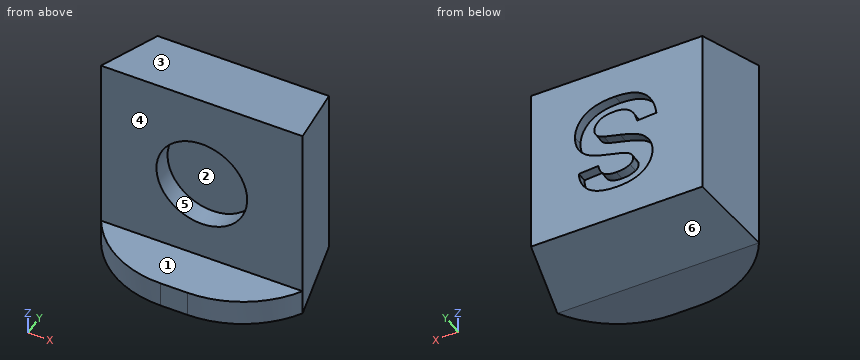
```python
from build123d import *

# Parameters (mm, degrees)
SKETCH1_W               = 8
SKETCH1_H               = 8
BOSS_EXTRUDE1_DEPTH     = 3
CUT_EXTRUDE1_DEPTH      = 12.704699911
CUT_EXTRUDE1_DEPTH_BACK = 12.704699911
CUT_EXTRUDE2_DEPTH      = 11
SKETCH4_R               = 1.8
CUT_EXTRUDE3_DEPTH      = 0.8
SKETCH5_W               = 8
SKETCH5_H               = 1
BOSS_EXTRUDE2_DEPTH     = 2
FILLET1_R               = 4
CUT_EXTRUDE4_DEPTH      = 0.4


with BuildPart() as part:
    # Sketch1 → Boss-Extrude1 (new body)
    with BuildSketch(Plane(origin=(0, 0, 0), x_dir=(1, 0, 0), z_dir=(0, 1, 0))):
        with Locations((4, 4)):
            Rectangle(SKETCH1_W, SKETCH1_H)
    extrude(amount=BOSS_EXTRUDE1_DEPTH)

    # Sketch2 → Cut-Extrude1 (cut, two sides: drawn at the far end of the back side and taken through both)
    with BuildSketch(Plane.XY.offset(-CUT_EXTRUDE1_DEPTH_BACK)):
        Polygon((0, 0), (0.6, 3), (0, 3), align=None)
        Polygon((8, 0), (7.4, 3), (8, 3), align=None)
    extrude(amount=CUT_EXTRUDE1_DEPTH + CUT_EXTRUDE1_DEPTH_BACK, mode=Mode.SUBTRACT)

    # Sketch3 → Cut-Extrude2 (cut)
    with BuildSketch(Plane(origin=(0, 0, 0), x_dir=(0, 0, -1), z_dir=(1, 0, 0))):
        Polygon((0, 0), (0.6, 3), (0, 3), align=None)
        Polygon((8, 3), (7.4, 3), (8, 0), align=None)
    extrude(amount=CUT_EXTRUDE2_DEPTH, mode=Mode.SUBTRACT)

    # Sketch4 → Cut-Extrude3 (cut)
    with BuildSketch(Plane.XZ):
        with Locations(Location((4, -3.75, 0), (0, 0, 270))):
            Circle(SKETCH4_R)
    extrude(amount=-CUT_EXTRUDE3_DEPTH, mode=Mode.SUBTRACT)

    # Sketch5 → Boss-Extrude2 (add)
    with BuildSketch(Plane.XZ):
        with Locations((4, -7.5)):
            Rectangle(SKETCH5_W, SKETCH5_H)
    extrude(amount=BOSS_EXTRUDE2_DEPTH)

    # Fillet1
    # the kernel refuses this fillet: 4 mm, written as the material it takes off along each edge
    with BuildSketch(Plane(origin=(8, -2, -16.660254038), x_dir=(0, 1, 0), z_dir=(0, 0, 1)), Plane(origin=(0, -2, 1.660254038), x_dir=(0, 1, 0), z_dir=(0, 0, -1))) as fillet1_piece_1:
        with BuildLine():
            CenterArc((4, 3.464101615), FILLET1_R, 180, 60)
            Line((0, 3.464101615), (-0.08, 3.464101615))
            Line((-0.08, 3.464101615), (-0.08, 0))
            Line((-0.08, 0), (0, -0.08))
            ThreePointArc((0, -0.08), (1, -0.08), (1.96, -0.069282032))
            Line((1.96, -0.069282032), (2, 0))
        make_face()
    extrude(amount=18.320508076, mode=Mode.SUBTRACT)

    # Sketch6 → Cut-Extrude4 (cut)
    with BuildSketch(Plane(origin=(0, 3, 0), x_dir=(1, 0, 0), z_dir=(0, 1, 0))):
        with BuildLine():
            Line((2.423916505, 3.336189685), (3.193147274, 3.387471736))
            add(Edge.make_bspline(
                [(3.193147274, 3.387471736), (3.199275518, 3.35528983), (3.211179242, 3.292778523), (3.237627081, 3.203691377), (3.266738832, 3.12063689), (3.30152897, 3.044505684), (3.339615284, 2.973890515), (3.38412658, 2.910803039), (3.431957638, 2.853229033), (3.485476185, 2.803236311), (3.543783948, 2.759451994), (3.607171876, 2.722111271), (3.674953108, 2.6897922), (3.747293374, 2.663178469), (3.824938253, 2.64331119), (3.907211345, 2.629176798), (3.994230643, 2.620125524), (4.053701404, 2.618879435), (4.084172915, 2.618240967)],
                knots=[0, 0, 0, 0, 1.204560339, 2.339781841, 3.415289417, 4.440034832, 5.416475564, 6.362424008, 7.275913008, 8.16578645, 9.05021719, 9.95355393, 10.867835453, 11.809845306, 12.784702352, 13.812224031, 14.87903166, 16, 16, 16, 16], degree=3))
            add(Edge.make_bspline(
                [(4.084172915, 2.618240967), (4.116246108, 2.618590883), (4.178630121, 2.619271489), (4.269031453, 2.627715), (4.353560804, 2.639811238), (4.431471751, 2.6589593), (4.504219207, 2.680373377), (4.569996427, 2.709670116), (4.629867843, 2.743459668), (4.683679212, 2.781802056), (4.730640445, 2.824326515), (4.771724475, 2.86872067), (4.807505951, 2.914025405), (4.835668504, 2.962251146), (4.858460082, 3.011447443), (4.873523718, 3.063081907), (4.883700097, 3.1159689), (4.884867031, 3.152113555), (4.885454967, 3.1703243)],
                knots=[0, 0, 0, 0, 1.417779877, 2.757654889, 4.012140507, 5.189587551, 6.302846416, 7.360586765, 8.365575446, 9.33904572, 10.275781718, 11.161696098, 12.012180333, 12.822428111, 13.625933072, 14.403138519, 15.195454004, 16, 16, 16, 16], degree=3))
            add(Edge.make_bspline(
                [(4.885454967, 3.1703243), (4.884733913, 3.193140887), (4.883323278, 3.237778199), (4.866340641, 3.301592127), (4.840872442, 3.360713887), (4.802526135, 3.41427025), (4.750979261, 3.463212961), (4.685226085, 3.508997669), (4.603431212, 3.550186), (4.542750055, 3.573160928), (4.510454967, 3.585388403)],
                knots=[0, 0, 0, 0, 0.90494901, 1.770400303, 2.607161909, 3.452839393, 4.36912122, 5.420987164, 6.627424851, 8, 8, 8, 8], degree=3))
            add(Edge.make_bspline(
                [(4.510454967, 3.585388403), (4.496597999, 3.590031937), (4.465588357, 3.600423411), (4.4126892, 3.615282239), (4.348970759, 3.633836968), (4.273512264, 3.654927379), (4.186339087, 3.676497317), (4.088424838, 3.703069034), (3.978575834, 3.729510064), (3.901725338, 3.749028827), (3.861416505, 3.759266608)],
                knots=[0, 0, 0, 0, 0.521821638, 1.167752076, 1.961721917, 2.891982557, 3.96540661, 5.168436773, 6.514817513, 8, 8, 8, 8], degree=3))
            add(Edge.make_bspline(
                [(3.861416505, 3.759266608), (3.808922441, 3.772373151), (3.707643728, 3.797660082), (3.563197092, 3.84264374), (3.430159098, 3.887337495), (3.309810688, 3.935832618), (3.200824367, 3.984842463), (3.104963023, 4.037807847), (3.02022624, 4.091978089), (2.970848149, 4.132466251), (2.947153685, 4.151894813)],
                knots=[0, 0, 0, 0, 1.293880989, 2.496331788, 3.617634808, 4.64976062, 5.598842568, 6.473791081, 7.267636666, 8, 8, 8, 8], degree=3))
            add(Edge.make_bspline(
                [(2.947153685, 4.151894813), (2.917769469, 4.179407128), (2.860158996, 4.233347566), (2.784323751, 4.321982057), (2.720601495, 4.415610216), (2.668151102, 4.513540942), (2.627765291, 4.616338017), (2.599140348, 4.723313361), (2.580613245, 4.834746169), (2.578722682, 4.91063455), (2.577762659, 4.949170454)],
                knots=[0, 0, 0, 0, 1.064429417, 2.086912298, 3.078678339, 4.055528992, 5.020032834, 5.993708893, 6.981211098, 8, 8, 8, 8], degree=3))
            add(Edge.make_bspline(
                [(2.577762659, 4.949170454), (2.579632311, 4.999035454), (2.583341142, 5.097952729), (2.617353538, 5.24334762), (2.670335558, 5.383642492), (2.731782138, 5.495041815), (2.790819043, 5.579315825), (2.839844896, 5.639790083), (2.893704531, 5.696388175), (2.953135712, 5.747729494), (3.015931612, 5.796821395), (3.084525186, 5.840415592), (3.156971597, 5.881478913), (3.261809808, 5.93015757), (3.404151332, 5.980885512), (3.589345301, 6.023645948), (3.790984862, 6.049350493), (3.930782191, 6.052503897), (4.003243428, 6.054138403)],
                knots=[0, 0, 0, 0, 1.180131776, 2.341029169, 3.518901375, 4.725685298, 5.343762192, 5.955650671, 6.568945152, 7.192346361, 7.815201106, 8.455999361, 9.116257477, 9.787318263, 11.192748436, 12.688084276, 14.283332633, 16, 16, 16, 16], degree=3))
            add(Edge.make_bspline(
                [(4.003243428, 6.054138403), (4.062574751, 6.053344994), (4.177972905, 6.051801831), (4.345255933, 6.036197125), (4.501507358, 6.011910245), (4.646178875, 5.977046542), (4.779337891, 5.930982439), (4.901500568, 5.876111383), (5.012563098, 5.81096567), (5.111173405, 5.735171454), (5.199025737, 5.651613191), (5.275662846, 5.560343317), (5.341377732, 5.462514514), (5.396594511, 5.358198276), (5.439956101, 5.246858263), (5.471803478, 5.128633406), (5.492867609, 5.003801978), (5.498147397, 4.918266237), (5.500839582, 4.874651223)],
                knots=[0, 0, 0, 0, 1.325124071, 2.577337985, 3.749592149, 4.855247722, 5.896868755, 6.892903601, 7.842551483, 8.766257401, 9.665194363, 10.546067736, 11.423174165, 12.293291263, 13.177512979, 14.086532529, 15.024315359, 16, 16, 16, 16], degree=3))
            Line((5.500839582, 4.874651223), (4.731608813, 4.823369172))
            add(Edge.make_bspline(
                [(4.731608813, 4.823369172), (4.727171315, 4.847490186), (4.718523093, 4.894499533), (4.699719489, 4.96182647), (4.678509937, 5.024096207), (4.653685255, 5.081308344), (4.623700039, 5.13243816), (4.591067506, 5.179094223), (4.554887475, 5.220654869), (4.51396201, 5.255982033), (4.469697485, 5.288128305), (4.419251527, 5.313894286), (4.364737876, 5.337799444), (4.30408262, 5.355770261), (4.238450559, 5.370025359), (4.167803464, 5.380593162), (4.091994892, 5.385752959), (4.039841388, 5.386885694), (4.012858813, 5.387471736)],
                knots=[0, 0, 0, 0, 1.151066407, 2.24330871, 3.278475654, 4.238599069, 5.165719782, 6.056502506, 6.909492653, 7.744782051, 8.590364415, 9.471203867, 10.39832458, 11.382154319, 12.435022857, 13.550631277, 14.73277401, 16, 16, 16, 16], degree=3))
            add(Edge.make_bspline(
                [(4.012858813, 5.387471736), (3.984804304, 5.386954358), (3.930223002, 5.385947775), (3.850683499, 5.379770524), (3.776069477, 5.368367912), (3.706014485, 5.353524542), (3.640612102, 5.333331162), (3.580000346, 5.308708643), (3.523901913, 5.279720359), (3.489695535, 5.256913378), (3.47279471, 5.245644813)],
                knots=[0, 0, 0, 0, 1.186678824, 2.308736671, 3.37120409, 4.377216403, 5.334874112, 6.262130804, 7.141346615, 8, 8, 8, 8], degree=3))
            add(Edge.make_bspline(
                [(3.47279471, 5.245644813), (3.453453136, 5.230251633), (3.415994509, 5.200439822), (3.3756811, 5.141243702), (3.351412335, 5.074383458), (3.348491314, 5.027102037), (3.346993428, 5.002856352)],
                knots=[0, 0, 0, 0, 1.037857257, 2.010007357, 2.979541333, 4, 4, 4, 4], degree=3))
            add(Edge.make_bspline(
                [(3.346993428, 5.002856352), (3.348218426, 4.980197149), (3.350631475, 4.935562125), (3.374970191, 4.872157107), (3.41239982, 4.813407798), (3.447371668, 4.781494404), (3.465583172, 4.764875582)],
                knots=[0, 0, 0, 0, 0.98538058, 1.941042925, 2.927803204, 4, 4, 4, 4], degree=3))
            add(Edge.make_bspline(
                [(3.465583172, 4.764875582), (3.480036346, 4.754089134), (3.512333176, 4.72998591), (3.571494566, 4.699348433), (3.642903916, 4.666166195), (3.728189187, 4.633726893), (3.826783574, 4.601347807), (3.938693075, 4.567540299), (4.063986517, 4.533278892), (4.199470233, 4.500098399), (4.337024364, 4.467483879), (4.46828848, 4.431827004), (4.590345232, 4.397064309), (4.702628677, 4.360627363), (4.805717615, 4.325156109), (4.899111277, 4.288724577), (4.98345094, 4.253244341), (5.081800337, 4.204456503), (5.193269487, 4.138371404), (5.310101731, 4.042305693), (5.413424942, 3.934321559), (5.485417809, 3.83249997), (5.534873142, 3.744930694), (5.566717158, 3.675127784), (5.59426473, 3.601573118), (5.616688379, 3.524185412), (5.632940128, 3.442855773), (5.646389397, 3.358205559), (5.653260877, 3.269531733), (5.654205671, 3.209062493), (5.654685736, 3.178337121)],
                knots=[0, 0, 0, 0, 0.511875881, 1.143829537, 1.88775736, 2.750598373, 3.734912702, 4.837306479, 6.073130119, 7.42648979, 8.801963576, 10.091065733, 11.292408984, 12.408830014, 13.446061236, 14.39066453, 15.257936293, 16.045629259, 17.510392066, 18.929669597, 20.331293837, 21.746891395, 22.460690638, 23.187651344, 23.925159671, 24.69163991, 25.474819891, 26.281170188, 27.126635539, 28, 28, 28, 28], degree=3))
            add(Edge.make_bspline(
                [(5.654685736, 3.178337121), (5.654025632, 3.150001459), (5.652714728, 3.093729578), (5.643553782, 3.010207902), (5.629386607, 2.928169417), (5.608414322, 2.847511277), (5.580592445, 2.768392154), (5.549267222, 2.689670139), (5.510096795, 2.613061996), (5.465515506, 2.538504273), (5.41634032, 2.466052922), (5.360615699, 2.3992182), (5.301614691, 2.335770341), (5.235567289, 2.279262071), (5.166552067, 2.225117883), (5.091412341, 2.177166881), (5.011908526, 2.133775469), (4.927537931, 2.095267608), (4.838001417, 2.061711489), (4.743415274, 2.031844209), (4.642927337, 2.007400135), (4.537375532, 1.986448484), (4.426373586, 1.970515295), (4.310060277, 1.959390224), (4.188409162, 1.953116354), (4.105547428, 1.952094705), (4.063339582, 1.9515743)],
                knots=[0, 0, 0, 0, 0.900570041, 1.788444861, 2.667795364, 3.545012114, 4.433698372, 5.332345486, 6.235991676, 7.164928091, 8.092777575, 9.015680987, 9.928493428, 10.842962589, 11.775229507, 12.714851019, 13.672254427, 14.652424454, 15.660007982, 16.709910502, 17.803296389, 18.945495772, 20.129342395, 21.366102753, 22.658353839, 24, 24, 24, 24], degree=3))
            add(Edge.make_bspline(
                [(4.063339582, 1.9515743), (4.002397965, 1.952569276), (3.883743193, 1.954506517), (3.711359118, 1.971846347), (3.549674268, 1.998386209), (3.398951853, 2.0369045), (3.259007654, 2.086353292), (3.129905498, 2.147263285), (3.012269836, 2.219998383), (2.90464369, 2.302794639), (2.808461007, 2.397160809), (2.721973345, 2.501141662), (2.646347447, 2.615673526), (2.58163302, 2.740577261), (2.526193974, 2.875177636), (2.480472858, 3.01953646), (2.446047261, 3.174342245), (2.431421007, 3.281307488), (2.423916505, 3.336189685)],
                knots=[0, 0, 0, 0, 1.217954099, 2.371385517, 3.459848295, 4.490682126, 5.476952527, 6.422732854, 7.338496285, 8.236688651, 9.131557988, 10.026443255, 10.935708282, 11.869506048, 12.834296687, 13.842423496, 14.892981177, 16, 16, 16, 16], degree=3))
        make_face()
    extrude(amount=-CUT_EXTRUDE4_DEPTH, mode=Mode.SUBTRACT)


solid = part.part
```
Model file for the job. Use its own axes, mm. Face numbers are marked on the shaded views. A direction names the side the tool comes from. Give positions to 0.01 mm unless a question says otherwise; leave off trailing zeros. Order: outer loops, then holes, each group sorted by start corner. A loop starts at its lowest first (then second) coordinate and runs counter-clockwise, first axis right, second up.
1) Wall check: probe 1 along Y at (x, z) = (2, -6.75); probe 2 along Y at (x, z) = (4.75, -3.5); probe 3 along X at (y, z) = (0.25, -3.75). Give the ranges that are in metal, low to high.
2) Saw through at C-C, the plane x = 2. Write the cut outline in (y, z).
3) 3-axis set-ups, long thin cutter, end or side, ignore diameter. For the marked faces 1, 2 and 3: which of +Z, -Z, +X, -X, +Y, -Y reach the whole face in a straight line?
4) Saw through at A-A, the plane x = 7.5. Write the cut outline in (y, z).
5) Mould opens along Z. For the marked faces 4, 5 and 6 say: +Z half, -Z half, draft (parallel to the pull), parting line (faces both ways), or undercut.
6) Pin check, flat tips, straight feed: pin 1 (1.5 mm diameter, centred on x = 3.5, z = -2.5, fed in from -Y); pin 2 (1 mm diameter, centred on x = 2, y = 1.5, fed in from -Z); pin 3 (3 mm diameter, centred on x = 6, y = 1, fed in from +Z). Stop position of each tip, or through.
7) Saw through at B-B, the plane z = -0.75. Write the cut outline in (x, y).
Computed:
1. probe 1: y = 0 to 3
1. probe 2: y = 0.8 to 2.6
1. probe 3: x = 0.05 to 2.2, 5.8 to 7.95
2. outline: (-1.72, -8) - (0, -8) - (3, -7.4) - (3, -0.6) - (0, 0) - (0, -7) - (-1.72, -7) - close
3. face 1: +Z, +X, -X, -Y
3. face 2: -Y
3. face 3: +Z, +X, -X, +Y
4. outline: (-0.69, -8) - (0, -8) - (2.5, -7.5) - (2.5, -0.5) - (0, 0) - (0, -7) - (-0.69, -7) - close
5. face 4: draft
5. face 5: undercut
5. face 6: -Z half
6. pin 1: stops at y = 0
6. pin 2: stops at z = -7.8
6. pin 3: stops at z = 0
7. outline: (0, 0) - (8, 0) - (7.4, 3) - (0.6, 3) - close
